Can you work these out from the model? Positions are in its coordinate system, mm. Give positions to 0.01 mm unless a question says otherwise; leave off trailing zeros. Loops run counter-clockwise (first coordinate to the right, second up) from the corner with the lowest first, then second, coordinate; pieces in that order, holes last. Notation, with made-up numbers: (-15, 78) - (31, 78) arc R24 cw to (31, 104) - close; hole circle Ø6 at (8.25, 59.5). An arc over 180 degrees is marked (long way). Write item = value, one per line.
from build123d import *

# Parameters (mm, degrees)
F0_R     = 3.81
F1_DEPTH = 82.55


with BuildPart() as f1:
    # F0 (on Top) → F1 (new body)
    with BuildSketch(Plane.XY):
        with BuildLine():
            ThreePointArc((20.308533, 33.133345), (0, 27.791465), (-20.308533, 33.133345))
            ThreePointArc((-20.308533, 33.133345), (-22.265361, 31.851354), (-24.141506, 30.453944))
            ThreePointArc((-24.141506, 30.453944), (-24.378061, 26.06285), (-28.775153, 26.119832))
            ThreePointArc((-28.775153, 26.119832), (-33.655479, 19.431), (-37.008014, 11.860098))
            ThreePointArc((-37.008014, 11.860098), (-34.76012, 8.080595), (-38.444642, 5.680186))
            ThreePointArc((-38.444642, 5.680186), (-38.716762, 3.356691), (-38.848585, 1.021033))
            ThreePointArc((-38.848585, 1.021033), (-24.068115, -13.895732), (-18.540052, -34.154378))
            ThreePointArc((-18.540052, -34.154378), (-16.451401, -35.208045), (-14.303136, -36.13413))
            ThreePointArc((-14.303136, -36.13413), (-10.382059, -34.143445), (-8.232861, -37.979929))
            ThreePointArc((-8.232861, -37.979929), (0, -38.862), (8.232861, -37.979929))
            ThreePointArc((8.232861, -37.979929), (10.382059, -34.143445), (14.303136, -36.13413))
            ThreePointArc((14.303136, -36.13413), (16.451401, -35.208045), (18.540052, -34.154378))
            ThreePointArc((18.540052, -34.154378), (24.068115, -13.895732), (38.848585, 1.021033))
            ThreePointArc((38.848585, 1.021033), (38.716762, 3.356691), (38.444642, 5.680186))
            ThreePointArc((38.444642, 5.680186), (34.76012, 8.080595), (37.008014, 11.860098))
            ThreePointArc((37.008014, 11.860098), (33.655479, 19.431), (28.775153, 26.119832))
            ThreePointArc((28.775153, 26.119832), (24.378061, 26.06285), (24.141506, 30.453944))
            ThreePointArc((24.141506, 30.453944), (22.265361, 31.851354), (20.308533, 33.133345))
        make_face()
        Circle(F0_R, mode=Mode.SUBTRACT)
        with BuildLine():
            ThreePointArc((-28.775153, 26.119832), (-24.378061, 26.06285), (-24.141506, 30.453944))
            ThreePointArc((-24.141506, 30.453944), (-26.546927, 28.381608), (-28.775153, 26.119832))
        make_face()
        with BuildLine():
            ThreePointArc((28.775153, 26.119832), (26.546927, 28.381608), (24.141506, 30.453944))
            ThreePointArc((24.141506, 30.453944), (24.378061, 26.06285), (28.775153, 26.119832))
        make_face()
        with BuildLine():
            ThreePointArc((-38.444642, 5.680186), (-34.76012, 8.080595), (-37.008014, 11.860098))
            ThreePointArc((-37.008014, 11.860098), (-37.852658, 8.799509), (-38.444642, 5.680186))
        make_face()
        with BuildLine():
            ThreePointArc((38.444642, 5.680186), (37.852658, 8.799509), (37.008014, 11.860098))
            ThreePointArc((37.008014, 11.860098), (34.76012, 8.080595), (38.444642, 5.680186))
        make_face()
        with BuildLine():
            ThreePointArc((-8.232861, -37.979929), (-10.382059, -34.143445), (-14.303136, -36.13413))
            ThreePointArc((-14.303136, -36.13413), (-11.30573, -37.181118), (-8.232861, -37.979929))
        make_face()
        with BuildLine():
            ThreePointArc((8.232861, -37.979929), (11.30573, -37.181118), (14.303136, -36.13413))
            ThreePointArc((14.303136, -36.13413), (10.382059, -34.143445), (8.232861, -37.979929))
        make_face()
    extrude(amount=F1_DEPTH)


solid = f1.part
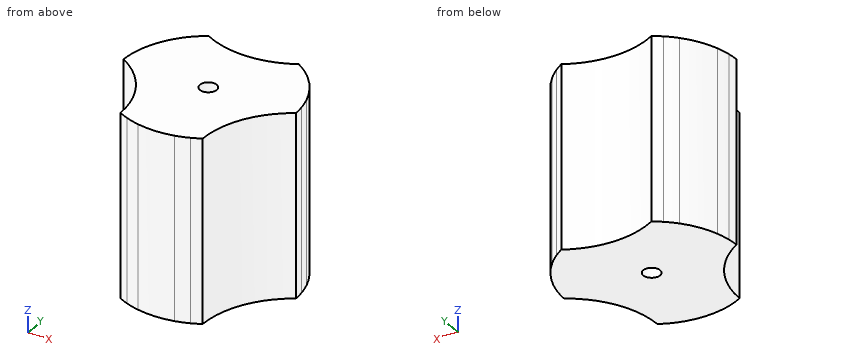
Q1. Imagine slicing it at D-D, the plane x = -32.5. Write out the boundary of the cut face in (y, z).
Output:
outline = (-3.59, 0) - (21.31, 0) - (21.31, 82.55) - (-3.59, 82.55) - close
Q2. Imagine slicing it at A-A, the plane x = 0. Write out the boundary of the cut face in (y, z), then the cut area to 3 significant figures.
Output:
outline = (-38.86, 0) - (-3.81, 0) - (-3.81, 82.55) - (-38.86, 82.55) - close; (3.81, 0) - (27.79, 0) - (27.79, 82.55) - (3.81, 82.55) - close
area = 4,870 mm2
Q3. Imagine slicing it at C-C, the plane y = -20.5. Write out the boundary of the cut face in (x, z).
Output:
outline = (-21, 0) - (21, 0) - (21, 82.55) - (-21, 82.55) - close
Q4. I need wall thicknesses on L1, parallel to Y at x = 0, z = 25; L2, parallel to X at y = -18, z = 62; L3, parallel to Y at x = -9.5, z = 32. Which ranges of each line are inside material? Lowest first, please.
Output:
L1 = -38.86 to -3.81, 3.81 to 27.79
L2 = -21.99 to 21.99
L3 = -37.68 to 28.9
Q5. For pin 1 (4 mm diameter, centred on x = 11, y = 11.5, fed in from -Z); pin 2 (3 mm diameter, centred on y = -25.5, z = 28, fed in from +X); pin 3 (2 mm diameter, centred on y = 18.5, z = 23, fed in from -X); pin 4 (5 mm diameter, centred on y = -9, z = 46.5, fed in from -X), each with a flat end and sliding along its axis, tell me the tip position at first contact or that it passes through.
Output:
pin_1 = 0
pin_2 = 19.9
pin_3 = -34.7
pin_4 = -29.52
